Here's the drawing with two shaded views (mm, measured from the low corner). I have some questions. A direction names the side the tool comes from. Give positions to 0.01 mm unless a question says otherwise; leave off trailing zeros. Write each loop counter-clockwise with the first axis right and the second up, starting at its lowest first coordinate (ties: lowest second). Pieces come first, ordered by that corner, then holes.
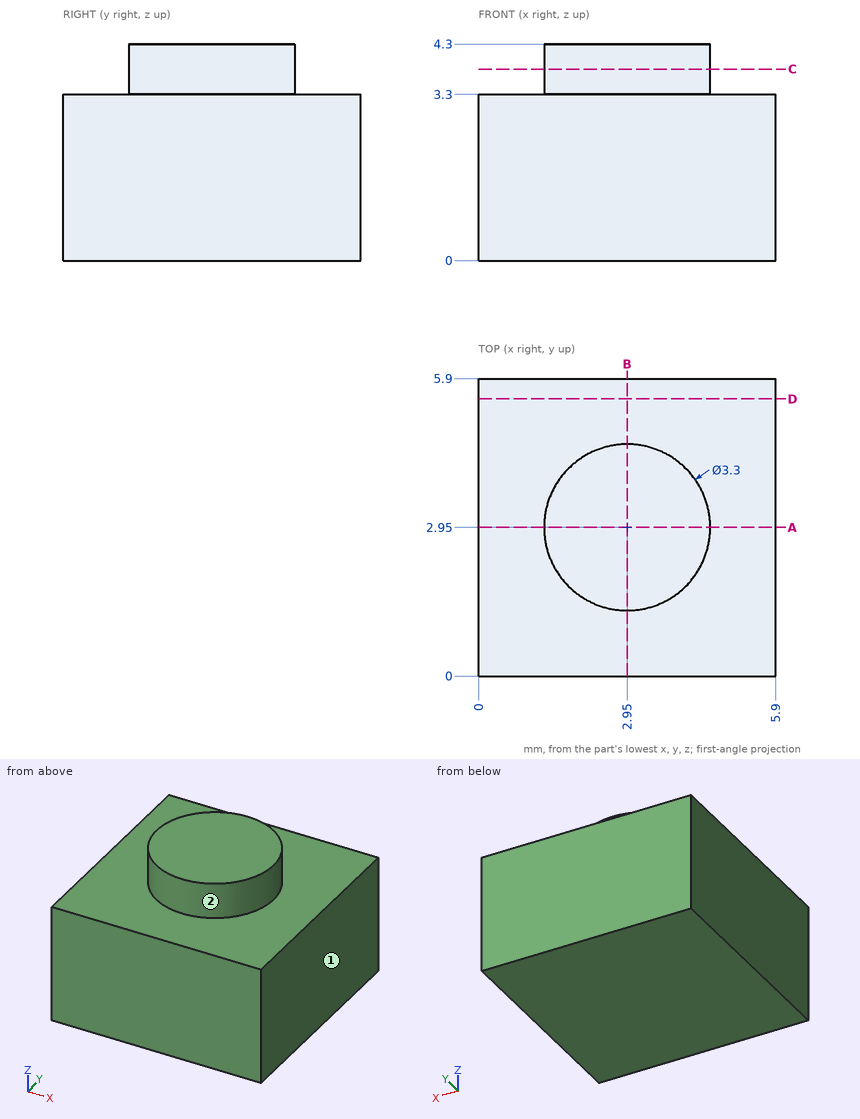
1) For the marked faces 1 and 2, which set-ups out of +Z, -Z, +X, -X, +Y, -Y let a thin tool reach every point of the face, with its end or its side?
Values follow:
face 1: +Z, -Z, +X, +Y, -Y
face 2: +Z
2) Please list where these lines run through material, in increasing order: L1, parallel to Z at x = 5.15, y = 0.45; L2, parallel to Y at x = 2.9, z = 3.5.
Values follow:
L1: z = 0 to 3.3
L2: y = 1.3 to 4.6
3) Suppose I cut it at D-D on y = 5.5. Write out the boundary of the cut face in (x, z), plus the area to 3 significant figures.
Values follow:
outline: (0, 0) - (5.9, 0) - (5.9, 3.3) - (0, 3.3) - close
area: 19.5 mm2
4) Suppose I cut it at C-C on z = 3.8. Write out the boundary of the cut face in (x, y).
Values follow:
outline: circle Ø3.3 at (2.95, 2.95)
5) Suppose I cut it at A-A on y = 2.95. Write out the boundary of the cut face in (x, z), plus the area to 3 significant figures.
Values follow:
outline: (0, 0) - (5.9, 0) - (5.9, 3.3) - (4.6, 3.3) - (4.6, 4.3) - (1.3, 4.3) - (1.3, 3.3) - (0, 3.3) - close
area: 22.8 mm2
